Part model, mm, in its own coordinate system. Face numbers are marked on the shaded views. A direction names the side the tool comes from. Round coordinates to 2 decimals unless told otherwise and drop trailing zeros. Write each loop counter-clockwise with the first axis right and the second up, starting at its lowest first coordinate (ties: lowest second). Pieces come first, ordered by that corner, then holes. Notation, with made-up numbers: M 19,76.5 L 29,76.5 A33 cw 29,112.5 Z; hole C 65.5,23 d1. An arc over 180 degrees is marked long. Use a Markdown table: item, result. Add a question column.
1) Slice it at B-B on x = 0. Write the cut outline in (y, z).
2) Slice it at D-D on x = -62. Write the cut outline in (y, z), plus the area to 3 significant figures.
3) Wall check: probe 1 along Y at (x, z) = (0.5, 45); probe 2 along X at (y, z) = (-49, 142); probe 3 along Y at (x, z) = (-14, 170). Give the ranges that are in metal, low to high.
4) Slice it at C-C on y = 0. Write the cut outline in (x, z).
5) Drop flat-ended pins along their axis: P1, Ø24.5, axis at x = 25.62, y = 45.29, coming from the +Z side; P2, Ø6, axis at x = -57, z = 31, coming from the -Y side; P3, Ø24, axis at y = 36.5, z = -35.5, coming from the -X side. Give the stop position or say it passes through.
6) Which spindle directions (+Z, -Z, +X, -X, +Y, -Y) get a long thin tool onto all of the face, cutting with end or side? Do the marked faces 1 and 2. Say none if no direction does.
7) Slice it at A-A on z = 106. Give the number of separate pieces and of enclosed holes in the cut face, plus the area to 3 significant figures.
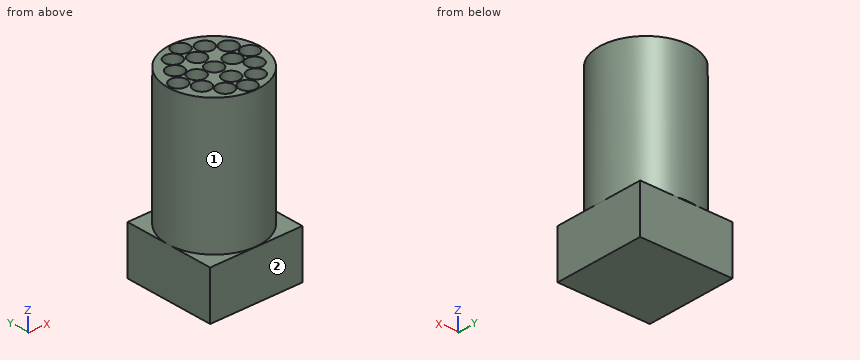
```python
from build123d import *

# Parameters (mm, degrees)
F0_R     = 75.661837
F1_DEPTH = 25.4
F2_R     = 75.661837
F2_R_2   = 13.687901
F3_DEPTH = 195.58
F4_W     = 151.870482
F4_H     = 150.282562
F5_DEPTH = 79.502


with BuildPart() as f1:
    # F0 (on Top) → F1 (new body)
    with BuildSketch(Plane.XY):
        Circle(F0_R)
    extrude(amount=F1_DEPTH)

    # F2 (on face) → F3 (join)
    with BuildSketch(Plane.XY.offset(25.4)):
        Circle(F2_R)
        with Locations((-25.131308, -47.922332)):
            Circle(F2_R_2, mode=Mode.SUBTRACT)
        with Locations((-42.732153, -25.166063)):
            Circle(F2_R_2, mode=Mode.SUBTRACT)
        with Locations((0, -60.893506)):
            Circle(F2_R_2, mode=Mode.SUBTRACT)
        with Locations((26.138142, -46.983935)):
            Circle(F2_R_2, mode=Mode.SUBTRACT)
        with Locations((0, -31.111687)):
            Circle(F2_R_2, mode=Mode.SUBTRACT)
        with Locations((44.296265, -24.778374)):
            Circle(F2_R_2, mode=Mode.SUBTRACT)
        with Locations((-58.921885, 0)):
            Circle(F2_R_2, mode=Mode.SUBTRACT)
        with Locations((-41.716155, 25.125945)):
            Circle(F2_R_2, mode=Mode.SUBTRACT)
        with Locations((-28.695317, 0)):
            Circle(F2_R_2, mode=Mode.SUBTRACT)
        with Locations((-24.919521, 47.710422)):
            Circle(F2_R_2, mode=Mode.SUBTRACT)
        Circle(F2_R_2, mode=Mode.SUBTRACT)
        with Locations((30.379288, 0)):
            Circle(F2_R_2, mode=Mode.SUBTRACT)
        with Locations((0, 30.979946)):
            Circle(F2_R_2, mode=Mode.SUBTRACT)
        with Locations((59.144725, 0)):
            Circle(F2_R_2, mode=Mode.SUBTRACT)
        with Locations((47.558412, 26.046298)):
            Circle(F2_R_2, mode=Mode.SUBTRACT)
        with Locations((25.620574, 45.285549)):
            Circle(F2_R_2, mode=Mode.SUBTRACT)
        with Locations((0, 61.093103)):
            Circle(F2_R_2, mode=Mode.SUBTRACT)
    extrude(amount=F3_DEPTH)

    # F4 (on Top) → F5 (join)
    with BuildSketch(Plane.XY):
        with Locations((0.422429, -1.071021)):
            Rectangle(F4_W, F4_H)
    extrude(amount=-F5_DEPTH)


solid = f1.part
```
Entries:
| question | item | result |
|---|---|---|
| 1 | outline | M -76.21,-79.5 L 74.07,-79.5 L 74.07,0 L 75.66,0 L 75.66,220.98 L 74.78,220.98 L 74.78,25.4 L 47.41,25.4 L 47.41,220.98 L 44.67,220.98 L 44.67,25.4 L 17.29,25.4 L 17.29,220.98 L 13.69,220.98 L 13.69,25.4 L -13.69,25.4 L -13.69,220.98 L -17.42,220.98 L -17.42,25.4 L -44.8,25.4 L -44.8,220.98 L -47.21,220.98 L -47.21,25.4 L -74.58,25.4 L -74.58,220.98 L -75.66,220.98 L -75.66,0 L -76.21,0 Z |
| 2 | outline | M -76.21,-79.5 L 74.07,-79.5 L 74.07,0 L 43.37,0 L 43.37,220.98 L 13.34,220.98 L 13.34,25.4 L -13.34,25.4 L -13.34,220.98 L -43.37,220.98 L -43.37,0 L -76.21,0 Z |
| 2 | area | 25,900 mm^2 |
| 3 | probe 1 | y = -75.66 to -74.57, -47.21 to -44.79, -17.43 to -13.68, 13.68 to 17.3, 44.66 to 47.41, 74.77 to 75.66 |
| 3 | probe 2 | x = -57.65 to -38.78, -11.49 to -6.78, 6.78 to 12.6, 39.68 to 57.65 |
| 3 | probe 3 | y = -74.36 to -55.89, -39.96 to 39.46, 55.96 to 74.36 |
| 4 | outline | M -75.66,0 L -75.51,0 L -75.51,-79.5 L 76.36,-79.5 L 76.36,0 L 75.66,0 L 75.66,220.98 L 72.83,220.98 L 72.83,25.4 L 45.46,25.4 L 45.46,220.98 L 44.07,220.98 L 44.07,25.4 L 16.69,25.4 L 16.69,220.98 L 13.69,220.98 L 13.69,25.4 L -13.69,25.4 L -13.69,220.98 L -15.01,220.98 L -15.01,25.4 L -42.38,25.4 L -42.38,220.98 L -45.23,220.98 L -45.23,25.4 L -72.61,25.4 L -72.61,220.98 L -75.66,220.98 Z |
| 5 | P1 | stops at z = 25.4 |
| 5 | P2 | stops at y = -53 |
| 5 | P3 | stops at x = -75.51 |
| 6 | face 1 | +Z |
| 6 | face 2 | +Z, -Z, +X, -X, -Y |
| 7 | separate pieces | 1 |
| 7 | enclosed holes | 17 |
| 7 | area | 7,980 mm^2 |
